Can you work these out from the model? Positions are in its coordinate system, mm. A direction names the side the tool comes from. Give positions to 0.01 mm unless a question says otherwise; leave off trailing zeros. Loops run counter-clockwise (first coordinate to the right, second up) from the corner with the lowest first, then second, coordinate; pieces in that order, holes last. Notation, with made-up numbers: (66, 39) - (88, 39) arc R21 ccw to (88, 48) - close; hole circle Ø7 at (-18.75, -12). An arc over 180 degrees is marked (long way). Write item = value, one per line.
from build123d import *

# Parameters (mm, degrees)
CHAMFER1_SIZE           = 0.5
CUT_EXTRUDE1_DEPTH      = 81.068720484
CUT_EXTRUDE1_DEPTH_BACK = 81.068720484
SKETCH2_W               = 110.89778328
SKETCH2_H               = 14.994305345


with BuildPart() as part:
    # Sketch1 → Revolve1 (revolve)
    with BuildSketch(Plane(origin=(0, 0, 0), x_dir=(1, 0, 0), z_dir=(0, 1, 0)), mode=Mode.PRIVATE) as revolve1_sk:
        Polygon((50.3, 19), (50.3, 14.1), (47, 14.1), (47, 0), (49, 0), (49, 2.5), (48, 2.5), (48, 7.5), (49, 7.5), (49, 10), (55, 10), (55, 12), (53, 12), (53, 19), align=None)
    revolve(revolve1_sk.sketch.rotate(Axis((0, 0, -69.169847328), (0, 0, 1)), 180), axis=Axis((0, 0, -69.169847328), (0, 0, 1)))

    # Chamfer1
    chamfer1_edges = [part.edges().sort_by_distance(p)[0] for p in [
        (49, 0, -10),
        (49, 0, -7.5),
        (48, 0, -7.5),
        (48, 0, -2.5),
        (49, 0, -2.5),
        (49, 0, 0),
        (50.3, 0, -19),
        (53, 0, -19),
    ]]
    chamfer(chamfer1_edges, length=CHAMFER1_SIZE - 0.0001)  # a hair under: the kernel refuses the full size

    # Sketch2 → Cut-Extrude1 (cut, two sides: drawn at the far end of the back side and taken through both)
    with BuildSketch(Plane(origin=(0, 0, 0), x_dir=(1, 0, 0), z_dir=(0, 1, 0)).offset(-CUT_EXTRUDE1_DEPTH_BACK)):
        with Locations((0.44889164, 2.502847328)):
            Rectangle(SKETCH2_W, SKETCH2_H)
    extrude(amount=CUT_EXTRUDE1_DEPTH + CUT_EXTRUDE1_DEPTH_BACK, mode=Mode.SUBTRACT)


solid = part.part
Q1. Which directions (+Z, -Z, +X, -X, +Y, -Y) give clear straight access to the entire face, cutting with the end or side of a thin tool? Please do faces 1 (the flat face through (15, -45, -14.1)), 2 (the cylindrical face through (-25.379, 48.794, -11.014)).
Output:
face_1 = -Z
face_2 = +Z, -Z
Q2. We'd pull the mould along X, two halves only. Please class faces 3 (the cylindrical face through (6.9, -52.55, -15.3)), 4 (the flat face through (27.5, -43, -19)), 5 (the cylindrical face through (6.12, -46.6, -12.02)): released by +X, released by -X, zero draft, split by the parting line, or undercut.
Output:
face_3 = split by the parting line
face_4 = zero draft
face_5 = undercut
Q3. I need wall thicknesses on L1, parallel to Y at x = 0, z = -16.7; L2, parallel to Y at x = 0, z = -11.8; L3, parallel to X at y = 4.5, z = -17.75. Which ranges of each line are inside material? Lowest first, please.
Output:
L1 = -53 to -50.3, 50.3 to 53
L2 = -55 to -47, 47 to 55
L3 = -52.81 to -50.1, 50.1 to 52.81
Q4. Imagine slicing it at A-A, the plane y = 0. Write out the boundary of the cut face in (x, z).
Output:
outline = (-55, -12) - (-53, -12) - (-53, -18.5) - (-52.5, -19) - (-50.8, -19) - (-50.3, -18.5) - (-50.3, -14.1) - (-47, -14.1) - (-47, -10) - (-55, -10) - close; (47, -14.1) - (50.3, -14.1) - (50.3, -18.5) - (50.8, -19) - (52.5, -19) - (53, -18.5) - (53, -12) - (55, -12) - (55, -10) - (47, -10) - close
Q5. For pin 1 (2 mm diameter, centred on x = 11, z = -17.5, fed in from +Y); pin 2 (1 mm diameter, centred on x = 42, z = -13, fed in from +Y); pin 3 (5 mm diameter, centred on x = -18.5, z = -17.5, fed in from +Y), each with a flat end and sliding along its axis, tell me the tip position at first contact or that it passes through.
Output:
pin_1 = 52.05
pin_2 = 32.97
pin_3 = 50.53
